Can you work these out from the model? Positions are in its coordinate system, mm. Face numbers are marked on the shaded views. A direction names the side the tool comes from. Give positions to 0.01 mm unless a question says otherwise; leave off trailing zeros. Loops run counter-clockwise (first coordinate to the right, second up) from the corner with the lowest first, then second, coordinate; pieces in that order, holes last. Notation, with made-up numbers: (11.5, 48.5) - (69.5, 48.5) arc R15 cw to (69.5, 58.5) - close; hole circle Ø6 at (-4.75, 74.25). An arc over 180 degrees is marked (long way). Answer as a JSON object with one key per item and string values.
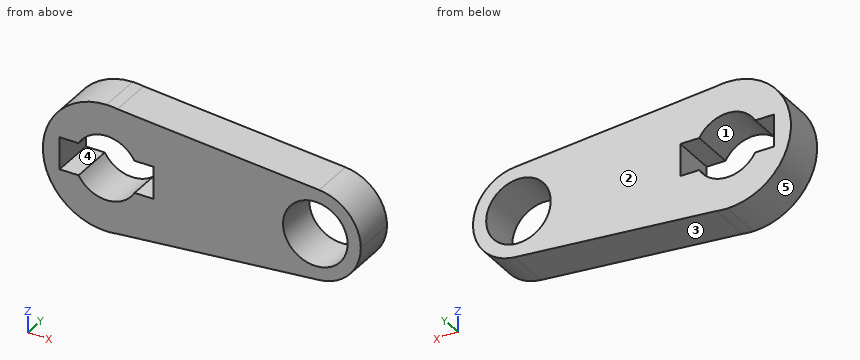
```python
from build123d import *

# Parameters (mm, degrees)
F0_R     = 10.16
F1_DEPTH = 13.716


with BuildPart() as f1:
    # F0 (on Front) → F1 (new body)
    with BuildSketch(Plane.XZ):
        with BuildLine():
            Line((3.440324, 19.740039), (0, 20.037589))
            ThreePointArc((0, 20.037589), (-20.037589, 0), (0, -20.037589))
            Line((0, -20.037589), (3.440324, -19.740039))
            ThreePointArc((3.440324, -19.740039), (15.336896, -12.895138), (20.037589, 0))
            ThreePointArc((20.037589, 0), (15.336896, 12.895138), (3.440324, 19.740039))
        make_face()
        with BuildLine():
            ThreePointArc((-8.798818, 5.08), (0, 10.16), (8.798818, 5.08))
            Line((8.798818, 5.08), (14.754587, 5.08))
            Line((14.754587, 5.08), (14.754587, -5.08))
            Line((14.754587, -5.08), (8.798818, -5.08))
            ThreePointArc((8.798818, -5.08), (0, -10.16), (-8.798818, -5.08))
            Line((-8.798818, -5.08), (-14.754587, -5.08))
            Line((-14.754587, -5.08), (-14.754587, 5.08))
            Line((-14.754587, 5.08), (-8.798818, 5.08))
        make_face(mode=Mode.SUBTRACT)
        with BuildLine():
            ThreePointArc((3.440324, 19.740039), (1.726584, 19.963063), (0, 20.037589))
            Line((0, 20.037589), (3.440324, 19.740039))
        make_face()
        with BuildLine():
            Line((3.440324, -19.740039), (0, -20.037589))
            ThreePointArc((0, -20.037589), (1.726584, -19.963063), (3.440324, -19.740039))
        make_face()
        with BuildLine():
            Line((66.929123, 14.248961), (3.440324, 19.740039))
            ThreePointArc((3.440324, 19.740039), (15.336896, 12.895138), (20.037589, 0))
            ThreePointArc((20.037589, 0), (15.336896, -12.895138), (3.440324, -19.740039))
            Line((3.440324, -19.740039), (66.929123, -14.248961))
            ThreePointArc((66.929123, -14.248961), (51.394591, 0), (66.929123, 14.248961))
        make_face()
        with BuildLine():
            ThreePointArc((79.998901, 0), (76.236606, 9.667626), (66.929123, 14.248961))
            ThreePointArc((66.929123, 14.248961), (51.394591, 0), (66.929123, -14.248961))
            ThreePointArc((66.929123, -14.248961), (76.236606, -9.667626), (79.998901, 0))
        make_face()
        with Locations((65.696746, 0)):
            Circle(F0_R, mode=Mode.SUBTRACT)
    extrude(amount=F1_DEPTH)


solid = f1.part
```
1) I'm going to push flat-ended pins straight in: P1, Ø3, axis at y = -9, z = 4, coming from the +X side; P2, Ø3, axis at x = -12.5, y = -3.5, coming from the -Z side; P3, Ø4, axis at y = -11, z = -4, coming from the -X side. Where does each tip first touch, or does it pass through?
Check sheet entries:
{"P1": "x = 79.78", "P2": "z = -16.75", "P3": "x = -19.94"}
2) Imagine slicing it at D-D on z = 8. Write out the boundary of the cut face in (x, y), and give its area (3 significant figures).
Check sheet entries:
{"outline": "(-18.37, -13.72) - (-6.26, -13.72) - (-6.26, 0) - (-18.37, 0) - close; (6.26, -13.72) - (59.43, -13.72) - (59.43, 0) - (6.26, 0) - close; (71.96, -13.72) - (77.55, -13.72) - (77.55, 0) - (71.96, 0) - close", "area": "972 mm2"}
3) If we mould it in two halves opening along X, with no side actions, what happens to the marked faces 3, 4 and 5? For each: released by +X, released by -X, zero draft, split by the parting line, or undercut.
Check sheet entries:
{"face 3": "released by +X", "face 4": "undercut", "face 5": "released by -X"}
4) I need wall thicknesses on L1, parallel to X at y = -2.5, z = -1.5; L2, parallel to X at y = -1.75, z = -6; L3, parallel to Z at x = -0.5, y = -2. Which ranges of each line are inside material? Lowest first, please.
Check sheet entries:
{"L1": "-19.98 to -14.75, 14.75 to 55.65, 75.75 to 79.92", "L2": "-19.12 to -8.2, 8.2 to 57.5, 73.9 to 78.68", "L3": "-20.03 to -10.15, 10.15 to 20.03"}
5) Imagine slicing it at A-A on y = -7.75. Write out the boundary of the cut face in (x, z).
Check sheet entries:
{"outline": "(0, -20.04) arc R20.04 ccw to (3.44, -19.74) - (66.93, -14.25) arc R14.3 ccw to (66.93, 14.25) - (3.44, 19.74) arc R20.04 ccw to (0, 20.04) arc R20.04 ccw to start; hole (-14.75, -5.08) - (-8.8, -5.08) arc R10.16 ccw to (8.8, -5.08) - (14.75, -5.08) - (14.75, 5.08) - (8.8, 5.08) arc R10.16 ccw to (-8.8, 5.08) - (-14.75, 5.08) - close; hole circle Ø20.32 at (65.7, 0)"}
6) Which directions (+Z, -Z, +X, -X, +Y, -Y) give clear straight access to the entire face, cutting with the end or side of a thin tool? Please do the marked faces 1 and 2.
Check sheet entries:
{"face 1": "+Y, -Y", "face 2": "+Z, -Z, +X, -X, +Y"}
7) Imagine slicing it at C-C on x = 69.5. Write out the boundary of the cut face in (y, z), and give its area (3 significant figures).
Check sheet entries:
{"outline": "(-13.72, -13.79) - (0, -13.79) - (0, -9.42) - (-13.72, -9.42) - close; (-13.72, 9.42) - (0, 9.42) - (0, 13.79) - (-13.72, 13.79) - close", "area": "120 mm2"}
8) Imagine slicing it at B-B on z = -6. Write out the boundary of the cut face in (x, y).
Check sheet entries:
{"outline": "(-19.12, -13.72) - (-8.2, -13.72) - (-8.2, 0) - (-19.12, 0) - close; (8.2, -13.72) - (57.5, -13.72) - (57.5, 0) - (8.2, 0) - close; (73.9, -13.72) - (78.68, -13.72) - (78.68, 0) - (73.9, 0) - close"}
